```python
from build123d import *

# Parameters (mm, degrees)
SKETCH1_R           = 2.5
BOSS_EXTRUDE1_DEPTH = 3


with BuildPart() as part:
    # Sketch1 → Boss-Extrude1 (new body)
    with BuildSketch(Plane(origin=(0, 0, 0), x_dir=(0, 0, -1), z_dir=(1, 0, 0))):
        with BuildLine():
            Line((-150, -20), (150, -20))
            ThreePointArc((150, -20), (170, 0), (150, 20))
            Line((150, 20), (-150, 20))
            ThreePointArc((-150, 20), (-170, 0), (-150, -20))
        make_face()
        with Locations((150, 0)):
            Circle(SKETCH1_R, mode=Mode.SUBTRACT)
        with Locations((-150, 0)):
            Circle(SKETCH1_R, mode=Mode.SUBTRACT)
        with Locations((90, 15)):
            Circle(SKETCH1_R, mode=Mode.SUBTRACT)
        with Locations((90, -15)):
            Circle(SKETCH1_R, mode=Mode.SUBTRACT)
        with Locations((-90, 15)):
            Circle(SKETCH1_R, mode=Mode.SUBTRACT)
        with Locations((-90, -15)):
            Circle(SKETCH1_R, mode=Mode.SUBTRACT)
        with Locations((0, 15)):
            Circle(SKETCH1_R, mode=Mode.SUBTRACT)
        with Locations((0, -15)):
            Circle(SKETCH1_R, mode=Mode.SUBTRACT)
    extrude(amount=BOSS_EXTRUDE1_DEPTH)


solid = part.part
```
For this review, take the finished solid that the model builds, in its own axes (mm). Coordinates: 2 decimals unless noted, no trailing zeros.
1. Add section A-A, the plane x = 1.05. Count the separate pieces of the cut face and the enclosed holes in it, then the cut area to 3 significant figures.
2. For line 1 (Y direction, x = 1.1, z = 90); line 2 (Z direction, x = 0.4, y = 14.5); line 3 (Y direction, x = 1.1, z = -92), list the stretches that pass through material, from the lowest coordinate up.
3. Insertion check: P1, Ø3, axis at y = 0, z = -150, coming from the -X side; P2, Ø6, axis at y = 16, z = 126, coming from the -X side. Each pin has a flat end and moves straight along its axis. Give the tip position at first contact, or say it passes through.
Result:
1. separate pieces: 1
1. enclosed holes: 8
1. area: 13,100 mm2
2. line 1: y = -20 to -17.5, -12.5 to 12.5, 17.5 to 20
2. line 2: z = -163.77 to -92.45, -87.55 to -2.45, 2.45 to 87.55, 92.45 to 163.77
2. line 3: y = -20 to -16.5, -13.5 to 13.5, 16.5 to 20
3. P1: passes through
3. P2: stops at x = 0
